Here's the drawing with two shaded views (mm, measured from the low corner). I have some questions. A direction names the side the tool comes from. Coordinates: 2 decimals unless noted, no trailing zeros. Loops run counter-clockwise (first coordinate to the right, second up) from the corner with the lowest first, then second, coordinate; pieces in that order, holes last. Notation, with made-up numbers: (75.25, -4.75) - (97.25, -4.75) arc R17 cw to (97.25, 2.25) - close; hole circle Ø8 at (8.5, 41.5). An arc over 180 degrees is marked (long way). One line per item, written item: value. Start each with the question number.
(1) If we section it at A-A on z = 9.5: Write out the boundary of the cut face in (x, y), then the cut area to 3 significant figures.
(2) If we section it at B-B on x = 2.25: Write out the boundary of the cut face in (y, z), then the cut area to 3 significant figures.
(3) If I drill on line 1 along Y through (x, z) = (15, 30.5); line 2 along Z through (x, y) = (3.25, 23.5); line 3 along Y through (x, z) = (4.05, 19.05), over which ranges is the centre line in solid material (lowest first)? Write a range as from..to.
(4) On a 3-axis mill with a long thin cutter (end or side, diameter ignored), from which of +Z, -Z, +X, -X, +Y, -Y can I reach the whole of each face in a straight line? I mean the marked faces 1, 2, 3 and 4. Say none if no direction works.
(5) If we mould it in two halves opening along Y, with no side actions, what happens to the marked faces 5, 6 and 7? For each: pulls with the +Y half, pulls with the -Y half, needs draft (parallel to the pull), parting line crosses it, or undercut.
(6) I'm going to push flat-ended pins straight in: P1, Ø3, axis at x = 4, y = 15.5, coming from the +Z side; P2, Ø5, axis at x = 9.5, y = 4.5, coming from the -Z side; P3, Ø2.5, axis at x = 15.875, y = 28.575, coming from the +Z side; P4, Ø6, axis at y = 11.5, z = 9, coming from the +X side. Where does each tip first touch, or does it pass through?
(7) If we section it at C-C on z = 26.5: Write out the boundary of the cut face in (x, y) (3 decimals).
(8) If we section it at D-D on x = 12.5: Write out the boundary of the cut face in (y, z), then the cut area to 3 significant figures.
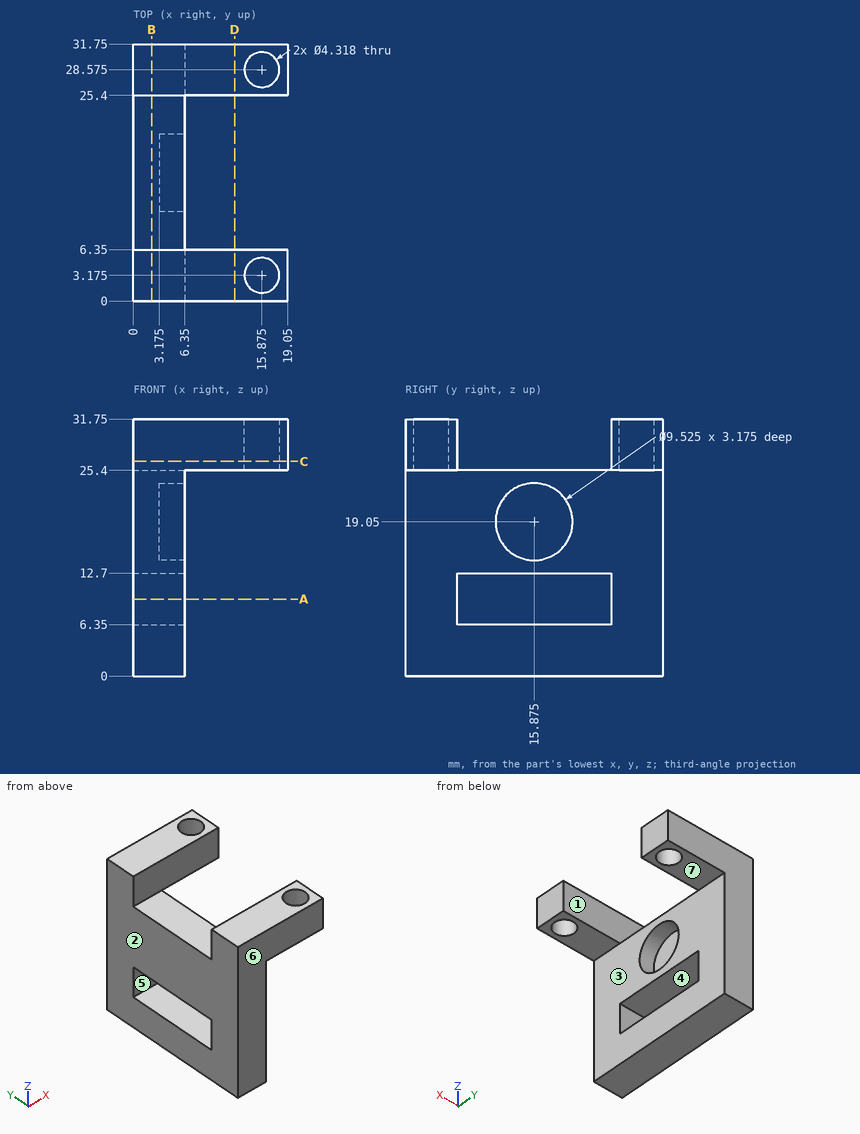
Values:
1. outline: (0, 0) - (6.35, 0) - (6.35, 6.35) - (0, 6.35) - close; (0, 25.4) - (6.35, 25.4) - (6.35, 31.75) - (0, 31.75) - close
1. area: 80.6 mm2
2. outline: (0, 0) - (31.75, 0) - (31.75, 31.75) - (25.4, 31.75) - (25.4, 25.4) - (6.35, 25.4) - (6.35, 31.75) - (0, 31.75) - close; hole (6.35, 6.35) - (25.4, 6.35) - (25.4, 12.7) - (6.35, 12.7) - close
2. area: 766 mm2
3. line 1: y = 0..1.2, 5.15..6.35, 25.4..26.6, 30.55..31.75
3. line 2: z = 0..6.35, 12.7..25.4
3. line 3: y = 0..11.11, 20.64..31.75
4. face 1: +Z, +X, -X
4. face 2: +Z, -Z, -X, +Y, -Y
4. face 3: -Z, +X, +Y, -Y
4. face 4: +X, -X
5. face 5: undercut
5. face 6: pulls with the -Y half
5. face 7: needs draft
6. P1: stops at z = 25.4
6. P2: stops at z = 25.4
6. P3: passes through
6. P4: stops at x = 6.35
7. outline: (0, 0) - (19.05, 0) - (19.05, 6.35) - (0, 6.35) - close; (0, 25.4) - (19.05, 25.4) - (19.05, 31.75) - (0, 31.75) - close; hole circle Ø4.318 at (15.875, 3.175); hole circle Ø4.318 at (15.875, 28.575)
8. outline: (0, 25.4) - (6.35, 25.4) - (6.35, 31.75) - (0, 31.75) - close; (25.4, 25.4) - (31.75, 25.4) - (31.75, 31.75) - (25.4, 31.75) - close
8. area: 80.6 mm2
